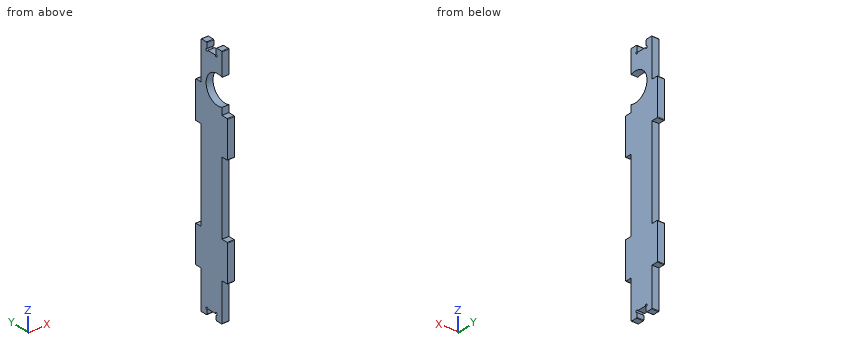
from build123d import *

# Parameters (mm, degrees)
BOSS_EXTRUDE1_DEPTH = 3


with BuildPart() as part:
    # Sketch3 → Boss-Extrude1 (new body)
    with BuildSketch(Plane(origin=(0, 0, 0), x_dir=(0, 0, -1), z_dir=(1, 0, 0))):
        with BuildLine():
            Line((73.486325357, 19.201934502), (89.186325357, 19.201934502))
            ThreePointArc((89.186325357, 19.201934502), (89.363102052, 19.128711197), (89.436325357, 18.951934502))
            Line((89.436325357, 18.951934502), (89.436325357, 16.201934502))
            Line((89.436325357, 16.201934502), (106.086325357, 16.201934502))
            ThreePointArc((106.086325357, 16.201934502), (106.263102052, 16.128711197), (106.336325357, 15.951934502))
            Line((106.336325357, 15.951934502), (106.336325357, 13.383184502))
            ThreePointArc((106.336325357, 13.383184502), (106.263102052, 13.206407807), (106.086325357, 13.133184502))
            Line((106.086325357, 13.133184502), (104.236325357, 13.133184502))
            ThreePointArc((104.236325357, 13.133184502), (103.382771966, 13.486737893), (103.736325357, 12.633184502))
            Line((103.736325357, 12.633184502), (103.736325357, 8.633184502))
            ThreePointArc((103.736325357, 8.633184502), (103.382771966, 7.779631112), (104.236325357, 8.133184502))
            Line((104.236325357, 8.133184502), (106.086325357, 8.133184502))
            ThreePointArc((106.086325357, 8.133184502), (106.263102052, 8.059961197), (106.336325357, 7.883184502))
            Line((106.336325357, 7.883184502), (106.336325357, 5.314434502))
            ThreePointArc((106.336325357, 5.314434502), (106.263102052, 5.137657807), (106.086325357, 5.064434502))
            Line((106.086325357, 5.064434502), (89.436325357, 5.064434502))
            Line((89.436325357, 5.064434502), (89.436325357, 2.314434502))
            ThreePointArc((89.436325357, 2.314434502), (89.363102052, 2.137657807), (89.186325357, 2.064434502))
            Line((89.186325357, 2.064434502), (73.486325357, 2.064434502))
            ThreePointArc((73.486325357, 2.064434502), (73.309548661, 2.137657807), (73.236325357, 2.314434502))
            Line((73.236325357, 2.314434502), (73.236325357, 5.064434502))
            Line((73.236325357, 5.064434502), (41.236325357, 5.064434502))
            Line((41.236325357, 5.064434502), (41.236325357, 2.314434502))
            ThreePointArc((41.236325357, 2.314434502), (41.163102052, 2.137657807), (40.986325357, 2.064434502))
            Line((40.986325357, 2.064434502), (25.286325357, 2.064434502))
            ThreePointArc((25.286325357, 2.064434502), (25.109548661, 2.137657807), (25.036325357, 2.314434502))
            Line((25.036325357, 2.314434502), (25.036325357, 5.064434502))
            Line((25.036325357, 5.064434502), (21.926862575, 5.064434502))
            ThreePointArc((21.926862575, 5.064434502), (16.086325357, 13.539434502), (10.245788138, 5.064434502))
            Line((10.245788138, 5.064434502), (0.386325357, 5.064434502))
            ThreePointArc((0.386325357, 5.064434502), (0.209548661, 5.137657807), (0.136325357, 5.314434502))
            Line((0.136325357, 5.314434502), (0.136325357, 7.883184502))
            ThreePointArc((0.136325357, 7.883184502), (0.209548661, 8.059961197), (0.386325357, 8.133184502))
            Line((0.386325357, 8.133184502), (2.636325357, 8.133184502))
            ThreePointArc((2.636325357, 8.133184502), (3.489878747, 7.779631112), (3.136325357, 8.633184502))
            Line((3.136325357, 8.633184502), (3.136325357, 12.633184502))
            ThreePointArc((3.136325357, 12.633184502), (3.489878747, 13.486737893), (2.636325357, 13.133184502))
            Line((2.636325357, 13.133184502), (0.386325357, 13.133184502))
            ThreePointArc((0.386325357, 13.133184502), (0.209548661, 13.206407807), (0.136325357, 13.383184502))
            Line((0.136325357, 13.383184502), (0.136325357, 15.951934502))
            ThreePointArc((0.136325357, 15.951934502), (0.209548661, 16.128711197), (0.386325357, 16.201934502))
            Line((0.386325357, 16.201934502), (17.036325357, 16.201934502))
            Line((17.036325357, 16.201934502), (17.036325357, 18.951934502))
            ThreePointArc((17.036325357, 18.951934502), (17.109548661, 19.128711197), (17.286325357, 19.201934502))
            Line((17.286325357, 19.201934502), (32.986325357, 19.201934502))
            ThreePointArc((32.986325357, 19.201934502), (33.163102052, 19.128711197), (33.236325357, 18.951934502))
            Line((33.236325357, 18.951934502), (33.236325357, 16.201934502))
            Line((33.236325357, 16.201934502), (73.236325357, 16.201934502))
            Line((73.236325357, 16.201934502), (73.236325357, 18.951934502))
            ThreePointArc((73.236325357, 18.951934502), (73.309548661, 19.128711197), (73.486325357, 19.201934502))
        make_face()
    extrude(amount=BOSS_EXTRUDE1_DEPTH)


solid = part.part
The listing builds one solid part. Answer for the finished solid, in the listing's coordinates (mm). Coordinates: 2 decimals unless noted, no trailing zeros. Write each loop counter-clockwise with the first axis right and the second up, starting at its lowest first coordinate (ties: lowest second). Pieces come first, ordered by that corner, then holes. Notation, with made-up numbers: (35.5, -1) - (59.5, -1) arc R23 ccw to (59.5, 9) - close; hole circle Ø3 at (42, 16). An arc over 180 degrees is marked (long way). Put each result on its own line as item: value.
1. The part is cut by section B-B on y = 11. Give the vertices of the cut face in (x, z), plus the area to 3 significant figures.
Answer sheet:
outline: (0, -103.74) - (3, -103.74) - (3, -21.12) - (0, -21.12) - close; (0, -11.06) - (3, -11.06) - (3, -3.14) - (0, -3.14) - close
area: 272 mm^2
2. Find the intervals of material crossed by line 1 along Z through (x, y) = (2.75, 3); line 2 along Z through (x, y) = (1.7, 18.25); line 3 along Y through (x, z) = (0.7, -8), in increasing order. Write a range as from..to.
Answer sheet:
line 1: z = -89.44..-73.24, -41.24..-25.04
line 2: z = -89.44..-73.24, -33.24..-17.04
line 3: y = 5.06..16.2
3. The part is cut by section C-C on z = -35.5. Give the vertices of the cut face in (x, y).
Answer sheet:
outline: (0, 2.06) - (3, 2.06) - (3, 16.2) - (0, 16.2) - close
4. The part is cut by section A-A on y = 3.25. Give the vertices of the cut face in (x, z).
Answer sheet:
outline: (0, -89.44) - (3, -89.44) - (3, -73.24) - (0, -73.24) - close; (0, -41.24) - (3, -41.24) - (3, -25.04) - (0, -25.04) - close
5. Flat-ended cylindrical pins translate along their axes: pin 1 Ø0.9 at (x, z) = (1.5, -23) entering from -Y; pin 2 Ø1.5 at (x, z) = (1.5, -59.5) entering from +Y; pin 3 Ø1.4 at (x, y) = (2, 17) entering from +Z; pin 4 Ø1.5 at (x, y) = (2, 5) entering from +Z. Find the tip coordinate at first contact, or state that the pin passes through.
Answer sheet:
pin 1: stops at y = 5.06
pin 2: stops at y = 16.2
pin 3: stops at z = -17.04
pin 4: stops at z = -0.14
6. The part is cut by section D-D on z = -97.5. Give the vertices of the cut face in (x, y).
Answer sheet:
outline: (0, 5.06) - (3, 5.06) - (3, 16.2) - (0, 16.2) - close
